Solid Edge part; units mm, degrees
sketch "Sketch1" plane through (0, 0, 0) normal (0, 0, 1) x (1, 0, 0)
  circle A0 centre (0, 0) radius 2
  line L0 (-20, 20) -> (-20, -20)
  line L1 (-20, -20) -> (20, -20)
  line L2 (20, -20) -> (20, 20)
  line L3 (20, 20) -> (-20, 20)
extrude "Protrusion1" add sketch "Sketch1" against normal blind 3
fillet "Redondeo_1" radius 10 1 edges at (-20, -20, -1.5)
sketch "Sketch2" plane through (0, 0, -3) normal (0, 0, -1) x (1, 0, 0)
  line L0 (-17, -20) -> (-20, -20)
  line L1 (-20, -20) -> (-20, 10)
  arc A0 (-20, 10) -> (-10, 20) centre (-10, 10) cw
  line L2 (-10, 20) -> (20, 20)
  line L3 (20, 17) -> (20, 20)
  line L4 (-10, 17) -> (20, 17)
  arc A1 (-17, 10) -> (-10, 17) centre (-10, 10) cw
  line L5 (-17, -20) -> (-17, 10)
extrude "ProtrusiónExtruida_2" add sketch "Sketch2" along normal blind 50
chamfer "Chaflán_1" distance 4 angle 45 3 edges at (5, -17, -3) (-14.9497, -14.9497, -3) (-17, 5, -3)
fillet "Redondeo_2" radius 3 1 edges at (20, 20, -1.5)
Design review of the part built by this model. Coordinates are the model's own, in mm. A direction names the side the tool comes from. Coordinates: 2 decimals unless noted, no trailing zeros. Order: outer loops, then holes, each group sorted by start corner. A loop starts at its lowest first (then second) coordinate and runs counter-clockwise, first axis right, second up. Notation, with made-up numbers: (43.25, 29.5) -> (95.25, 29.5) arc R34 cw to (95.25, 60.5) -> close; hole circle Ø10 at (-30.75, 66). An arc over 180 degrees is marked (long way). One line per item, written item: value. Start each with the question number.
Q1. Insertion check: pin 1 Ø9 at (x, z) = (-0.5, -30.5) entering from +Y; pin 2 Ø3 at (y, z) = (-11, -30.5) entering from +X; pin 3 Ø4 at (x, y) = (-6.5, 2.5) entering from -Z. Each pin has a flat end and moves straight along its axis. Give the tip position at first contact, or say it passes through.
Q2. Mouldability with a two-part tool opening along X and no side actions: class faces 1 (the cylindrical face through (-16.99, -17.15, -26.87)), 2 (the flat face through (3, 4, -3)), 3 (the cylindrical face through (0, -2, -1)), 4 (the cylindrical face through (19.1, 19.14, -1.52)) as pulls with the +X half, pulls with the -X half, needs draft (parallel to the pull), parting line crosses it, or undercut.
Q3. Take a section at D-D, the plane x = 12. State the section outline as (y, z) points.
Q4. Tool access review of faces 5 (the flat face through (4, 0, 0)), 6 (the flat face through (5, -15, -5)): name each direction out of +Z, -Z, +X, -X, +Y, -Y from which nothing blocks a thin tool from reaching the whole face with its end or side.
Q5. Take a section at A-A, the plane y = 0. State the section outline as (x, z) points.
Q6. Take a section at C-C, the plane z = -5.5. State the section outline as (x, y) points.
Q7. For probe 1 along Y at (x, z) = (0, -1.85); probe 2 along X at (y, z) = (14.5, -28); probe 3 along Z at (x, y) = (-11.5, 13), list the stretches that pass through material, from the lowest coordinate up.
Values follow:
1. pin 1: stops at y = -17
1. pin 2: stops at x = -16.54
1. pin 3: stops at z = -3
2. face 1: pulls with the -X half
2. face 2: needs draft
2. face 3: undercut
2. face 4: pulls with the +X half
3. outline: (-20, -53) -> (-17, -53) -> (-17, -7) -> (-13, -3) -> (20, -3) -> (20, 0) -> (-20, 0) -> close
4. face 5: +Z, +X, -X, +Y, -Y
4. face 6: -Z, +X, +Y
5. outline: (-20, -53) -> (-17, -53) -> (-17, -7) -> (-13, -3) -> (-2, -3) -> (-2, 0) -> (-20, 0) -> close; (2, -3) -> (20, -3) -> (20, 0) -> (2, 0) -> close
6. outline: (-20, -10) arc R10 ccw to (-10, -20) -> (20, -20) -> (20, -15.5) -> (-10, -15.5) arc R5.5 cw to (-15.5, -10) -> (-15.5, 20) -> (-20, 20) -> close
7. probe 1: y = -20 to -2, 2 to 20
7. probe 2: x = -20 to -17
7. probe 3: z = -3 to 0
